from build123d import *

# Parameters (mm, degrees)
BOSS_EXTRUDE1_DEPTH = 4


with BuildPart() as part:
    # Sketch1 → Boss-Extrude1 (new body)
    with BuildSketch(Plane.XY):
        with BuildLine():
            ThreePointArc((7.884132017, -3.176548808), (3.33142336, 7.819950025), (-7.75272605, 3.485001979))
            ThreePointArc((-7.75272605, 3.485001979), (-14.196448744, -39.008497905), (2.279937241, -78.704187839))
            ThreePointArc((2.279937241, -78.704187839), (10.324774467, -79.994584542), (12.238678661, -72.074893868))
            ThreePointArc((12.238678661, -72.074893868), (2.247032536, -38.119609121), (7.884132017, -3.176548808))
        make_face()
        with BuildLine():
            Line((-1.85, -2.04), (-1.85, 2.04))
            ThreePointArc((-1.85, 2.04), (0, 2.753924472), (1.85, 2.04))
            Line((1.85, 2.04), (1.85, -2.04))
            ThreePointArc((1.85, -2.04), (0, -2.753924472), (-1.85, -2.04))
        make_face(mode=Mode.SUBTRACT)
    extrude(amount=BOSS_EXTRUDE1_DEPTH)


solid = part.part
Geometry check sheet. Reference: the model listing, model coordinates, mm. A direction names the side the tool comes from. Give positions to 0.01 mm unless a question says otherwise; leave off trailing zeros. Loops run counter-clockwise (first coordinate to the right, second up) from the corner with the lowest first, then second, coordinate; pieces in that order, holes last. Notation, with made-up numbers: (32, 80) -> (36, 80) arc R20 ccw to (36, 85) -> close; hole circle Ø5 at (16.5, 21). An arc over 180 degrees is marked (long way). Answer in a Markdown table with one row per item. Add a question column.
1) Cross-section at B-B on x = 0. Record the boundary of the cut face in (y, z), and give its area (3 significant figures).
2) Cross-section at C-C on z = 2.75. Record the boundary of the cut face in (x, y) (3 decimals), and give its area (3 significant figures).
3) Cross-section at A-A on y = 0. Record the boundary of the cut face in (x, z), and give its area (3 significant figures).
4) Set-up check for faces 4 (the face through (-1.85, 0, 2)), 5 (the face through (-14.27, -38.4, 1.97)): record each of +Z, -Z, +X, -X, +Y, -Y from which the full face is reachable in a straight line by a thin tool's end or side.
5) Gauge pin test, flat end, axial feed: P1, Ø1.2, axis at y = -0.5, z = 1.5, coming from the +X side. Record the tip position at first contact, or that the pin passes through.
6) Draft check along X on faces 1 (the face through (10.22, -80.063, 1.972)), 2 (the face through (0.028, -2.754, 1.972)), 3 (the face through (-1, -36, 0)). Enter one of: pulls with the +X half, pulls with the -X half, needs draft (parallel to the pull), parting line crosses it, or undercut.
7) Material ranges on probe 1 along Y at (x, z) = (1.75, 3.65); probe 2 along Y at (x, z) = (-0.75, 3.8); probe 3 along Y at (x, z) = (-8.75, 1.5), recorded low to high. Write a range as from..to.
8) Cross-section at D-D on y = -16.5. Record the boundary of the cut face in (x, z).
Outcome:
| question | item | result |
|---|---|---|
| 1 | outline | (-75.65, 0) -> (-2.75, 0) -> (-2.75, 4) -> (-75.65, 4) -> close; (2.75, 0) -> (8.5, 0) -> (8.5, 4) -> (2.75, 4) -> close |
| 1 | area | 315 mm^2 |
| 2 | outline | (-7.753, 3.485) arc R80 ccw to (2.28, -78.704) arc R6 ccw to (12.239, -72.075) arc R80 cw to (7.884, -3.177) arc R8.5 ccw to start; hole (-1.85, -2.04) arc R2.754 ccw to (1.85, -2.04) -> (1.85, 2.04) arc R2.754 ccw to (-1.85, 2.04) -> close |
| 2 | area | 1,390 mm^2 |
| 3 | outline | (-9.22, 0) -> (-1.85, 0) -> (-1.85, 4) -> (-9.22, 4) -> close; (1.85, 0) -> (8.5, 0) -> (8.5, 4) -> (1.85, 4) -> close |
| 3 | area | 56.1 mm^2 |
| 4 | face 4 | +Z, -Z |
| 4 | face 5 | +Z, -Z, -X |
| 5 | P1 | stops at x = 8.5 |
| 6 | face 1 | parting line crosses it |
| 6 | face 2 | undercut |
| 6 | face 3 | needs draft |
| 7 | probe 1 | y = -78.02..-2.13, 2.13..8.32 |
| 7 | probe 2 | y = -74.58..-2.65, 2.65..8.47 |
| 7 | probe 3 | y = -59.8..1.17 |
| 8 | outline | (-13.75, 0) -> (3.82, 0) -> (3.82, 4) -> (-13.75, 4) -> close |
